from build123d import *

# Parameters (mm, degrees)
F1_DEPTH = 25.4


with BuildPart() as f1:
    # F0 (on Top) → F1 (new body)
    with BuildSketch(Plane.XY):
        Polygon((-24.0792, 34.290001), (-60.350399, 34.290001), (-67.761458, 24.655646), (-67.761458, -11.726021), (-60.350399, -23.129791), (48.551362, -23.129791), (52.7304, -13.2588), (52.7304, -5.9436), (48.1584, 0), (43.2816, 4.1148), (43.2816, -3.5052), (48.1584, -8.382), (45.998619, -10.54178), (-3.432985, -10.54178), align=None)
        Polygon((-57.912, -19.534851), (-63.144549, 0), (-57.912, 0), (-54.045353, -16.82521), (38.240661, -16.736207), (-14.135674, -14.026972), (-25.280462, -0.006108), (-18.946942, 0), (-9.141184, -12.336277), (43.86873, -12.336277), (46.566502, -18.194295), (43.86873, -19.43669), align=None, mode=Mode.SUBTRACT)
        Polygon((-62.263511, 16.462522), (-60.232367, 21.044958), (-55.59146, 21.044958), (-53.481128, 16.462522), (-50.370198, 21.045681), (-45.148745, 21.045681), (-43.03808, 16.462522), (-53.481128, 5.661911), align=None, mode=Mode.SUBTRACT)
        Polygon((-33.659617, 13.975172), (-34.229498, 18.544318), (-20.831046, 18.55724), (-20.826635, 13.983417), (-25.107411, 13.979289), (-25.100542, 6.856575), (-29.384067, 6.852444), (-29.39094, 13.979289), align=None, mode=Mode.SUBTRACT)
    extrude(amount=F1_DEPTH)


solid = f1.part
Could you check a few things on this model? Use its own coordinates, in mm. A direction names the side the tool comes from. Give positions to 0.01 mm unless a question says otherwise; leave off trailing zeros. Order: outer loops, then holes, each group sorted by start corner. A loop starts at its lowest first (then second) coordinate and runs counter-clockwise, first axis right, second up. Notation, with made-up numbers: (36, 80) -> (72, 80) arc R19 ccw to (72, 98) -> close; hole circle Ø3 at (-29.5, 64). An arc over 180 degrees is marked (long way). Return JSON: item names as keys, results as strings.
1. For pin 1 Ø7.5 at (x, z) = (22, 16.5) entering from +Y; pin 2 Ø10 at (x, y) = (-49, 20.5) entering from -Z; pin 3 Ø4 at (y, z) = (5, 5.5) entering from +X; pin 4 Ø2 at (y, z) = (-15, 21) entering from -X, each with a flat end and sliding along its axis, tell me the tip position at first contact or that it passes through.
Answer list:
{"pin 1": "stops at y = -10.54", "pin 2": "stops at z = 0", "pin 3": "stops at x = 44.6", "pin 4": "stops at x = -66.28"}
2. Imagine slicing it at B-B on y = 2.5. List the corners of the cut face in (x, z) for me.
Answer list:
{"outline": "(-67.76, 0) -> (-9.44, 0) -> (-9.44, 25.4) -> (-67.76, 25.4) -> close; (43.28, 0) -> (45.2, 0) -> (45.2, 25.4) -> (43.28, 25.4) -> close"}
3. Imagine slicing it at D-D on x = -16. List the corners of the cut face in (y, z) for me, then the cut area to 3 significant figures.
Answer list:
{"outline": "(-23.13, 0) -> (-19.49, 0) -> (-19.49, 25.4) -> (-23.13, 25.4) -> close; (-16.79, 0) -> (-11.68, 0) -> (-11.68, 25.4) -> (-16.79, 25.4) -> close; (-3.71, 0) -> (16.75, 0) -> (16.75, 25.4) -> (-3.71, 25.4) -> close", "area": "742 mm2"}
4. I need wall thicknesses on line 1 (Y direction, x = -38, z = 14.5); line 2 (Y direction, x = 9, z = 15.5); line 3 (X direction, y = -10, z = 13.5). Which ranges of each line are inside material? Lowest first, please. Write a range as from..to.
Answer list:
{"line 1": "y = -23.13..-19.52, -16.81..34.29", "line 2": "y = -23.13..-19.47, -16.76..-15.22, -12.34..-10.54", "line 3": "x = -67.76..-60.47, -55.61..-17.34, -11..-3.68, 46.54..52.73"}
5. Imagine slicing it at A-A on x = 14. List the corners of the cut face in (y, z) for me, then the cut area to 3 significant figures.
Answer list:
{"outline": "(-23.13, 0) -> (-19.47, 0) -> (-19.47, 25.4) -> (-23.13, 25.4) -> close; (-16.76, 0) -> (-15.48, 0) -> (-15.48, 25.4) -> (-16.76, 25.4) -> close; (-12.34, 0) -> (-10.54, 0) -> (-10.54, 25.4) -> (-12.34, 25.4) -> close", "area": "171 mm2"}
6. Thinking about a two-plate mould opening in Y: for faces 4 (the flat face through (-67.761, 7, 13)), 5 (the flat face through (-64.108, -17.348, 12.522)), 6 (the flat face through (-44.11, 18.79, 12.52)), which applies, pulls with the +Y half, pulls with the -Y half, needs draft (parallel to the pull), parting line crosses it, or undercut?
Answer list:
{"face 4": "needs draft", "face 5": "pulls with the -Y half", "face 6": "undercut"}
7. Imagine slicing it at C-C on z = 6.25. Give the number of separate pieces and of enclosed holes in the cut face, then the cut area to 3 significant figures.
Answer list:
{"separate pieces": "1", "enclosed holes": "3", "area": "3,020 mm2"}
8. On a 3-axis mill with a long thin cutter (end or side, diameter ignored), from which of +Z, -Z, +X, -X, +Y, -Y can I reach the whole of each face in a straight line? I mean faces 1 (the flat face through (-61, 0, 13)), 2 (the flat face through (43.282, 0, 13)), 3 (the flat face through (-64.004, 29.54, 12.522)). Say none if no direction works.
Answer list:
{"face 1": "+Z, -Z", "face 2": "+Z, -Z, +Y", "face 3": "+Z, -Z, -X, +Y"}
